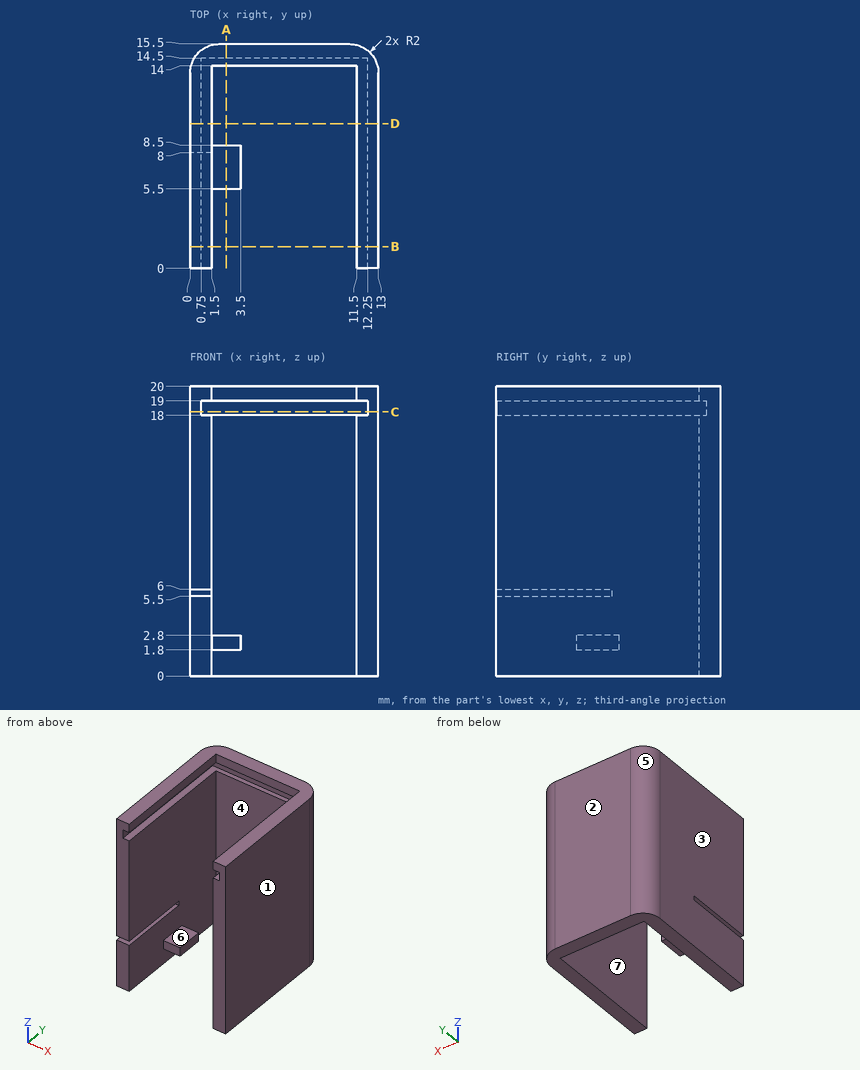
Verification items for this drawing (mm, ordinates from the low corner). A direction names the side the tool comes from. Give positions to 0.01 mm unless a question says otherwise; leave off trailing zeros. Loops run counter-clockwise (first coordinate to the right, second up) from the corner with the lowest first, then second, coordinate; pieces in that order, holes last. Notation, with made-up numbers: M 2,-20 L 33,-20 A10 ccw 33,-2 Z; hole C -17.75,-21.75 d6. An arc over 180 degrees is marked long. Answer in a Markdown table with one row per item.
1) Thickness scan on line 1 (X direction, y = 2, z = 16); line 2 (Y direction, x = 7, z = 11.5); line 3 (Y direction, x = 12.25, z = 16). Record the ranges inside material, lowest first.
Solutions:
| item | result |
|---|---|
| line 1 | x = 0 to 1.5, 11.5 to 13 |
| line 2 | y = 14 to 15.5 |
| line 3 | y = 0 to 15.06 |
2) Cross-section at B-B (y = 1.5). Enter the section's corners in (x, z), plus the area to 4 significant figures.
Solutions:
| item | result |
|---|---|
| outline | M 0,0 L 1.5,0 L 1.5,5.5 L 0,5.5 Z; M 0,6 L 1.5,6 L 1.5,18 L 0.75,18 L 0.75,19 L 1.5,19 L 1.5,20 L 0,20 Z; M 11.5,0 L 13,0 L 13,20 L 11.5,20 L 11.5,19 L 12.25,19 L 12.25,18 L 11.5,18 Z |
| area | 57.75 mm^2 |
3) Cross-section at D-D (y = 10). Enter the section's corners in (x, z), plus the area to 3 significant figures.
Solutions:
| item | result |
|---|---|
| outline | M 0,0 L 1.5,0 L 1.5,18 L 0.75,18 L 0.75,19 L 1.5,19 L 1.5,20 L 0,20 Z; M 11.5,0 L 13,0 L 13,20 L 11.5,20 L 11.5,19 L 12.25,19 L 12.25,18 L 11.5,18 Z |
| area | 58.5 mm^2 |
4) Tool access check on the marked faces 5, 6 and 7. Record the directions out of +Z, -Z, +X, -X, +Y, -Y that give a thin tool (end or side, any length) a straight path to the whole face; none if there is none.
Solutions:
| item | result |
|---|---|
| face 5 | +Z, -Z, -X, +Y |
| face 6 | +Z, -Y |
| face 7 | +Z, -Z, -Y |
5) Cross-section at A-A (x = 2.5). Enter the section's corners in (y, z), plus the area to 3 significant figures.
Solutions:
| item | result |
|---|---|
| outline | M 5.5,1.8 L 8.5,1.8 L 8.5,2.8 L 5.5,2.8 Z; M 14,0 L 15.5,0 L 15.5,20 L 14,20 L 14,19 L 14.5,19 L 14.5,18 L 14,18 Z |
| area | 32.5 mm^2 |
6) Mould release check, pull along X, two halves, no side actions. Record for the marked faces 1, 2, 3 and 4: released by +X, released by -X, zero draft, split by the parting line, or undercut.
Solutions:
| item | result |
|---|---|
| face 1 | released by +X |
| face 2 | zero draft |
| face 3 | released by -X |
| face 4 | undercut |
7) Cross-section at C-C (z = 18.25). Enter the section's corners in (x, y), plus the area to 3 significant figures.
Solutions:
| item | result |
|---|---|
| outline | M 0,0 L 0.75,0 L 0.75,14.5 L 12.25,14.5 L 12.25,0 L 13,0 L 13,13.5 A2 ccw 11,15.5 L 2,15.5 A2 ccw 0,13.5 Z |
| area | 33.0 mm^2 |
8) Depth check by flat-ended pin: pin 1 (0.8 mm diameter, centred on x = 3, z = 2, fed in from -Y); pin 2 (5 mm diameter, centred on x = 4.5, z = 10.5, fed in from -Y); pin 3 (0.5 mm diameter, centred on x = 6.5, z = 18.5, fed in from -Y). Enter the tip coordinate at first touch or a pass-through.
Solutions:
| item | result |
|---|---|
| pin 1 | stops at y = 5.5 |
| pin 2 | stops at y = 14 |
| pin 3 | stops at y = 14.5 |
